Geometry: final body of the model. Coordinates: model frame, mm. Round coordinates to 2 decimals unless told otherwise and drop trailing zeros. Write each loop counter-clockwise with the first axis right and the second up, starting at its lowest first coordinate (ties: lowest second). Pieces come first, ordered by that corner, then holes. Notation, with made-up numbers: M 81.5,78.5 L 88.5,78.5 A34 ccw 88.5,117.5 Z; hole C -38,-33.5 d5. An arc over 180 degrees is marked long. Use one line per item in the form item = value. Start each with the question number.
from build123d import *

# Parameters (mm, degrees)
SKETCH1_R           = 1.5
SKETCH1_R_2         = 2
SKETCH1_W           = 10
SKETCH1_H           = 5
BOSS_EXTRUDE2_DEPTH = 5


with BuildPart() as part:
    # Sketch1 → Boss-Extrude2 (new body)
    with BuildSketch(Plane.XY):
        with BuildLine():
            Line((-126.904376013, 20), (173.095623987, 20))
            ThreePointArc((173.095623987, 20), (193.095623987, 0), (173.095623987, -20))
            Line((173.095623987, -20), (-126.904376013, -20))
            ThreePointArc((-126.904376013, -20), (-146.904376013, 0), (-126.904376013, 20))
        make_face()
        with Locations((-126.904376013, 0)):
            Circle(SKETCH1_R, mode=Mode.SUBTRACT)
        with Locations((173.095623987, 0)):
            Circle(SKETCH1_R_2, mode=Mode.SUBTRACT)
        with Locations((-26.904376013, 0)):
            Circle(SKETCH1_R, mode=Mode.SUBTRACT)
        with Locations((28.095623987, 12.5)):
            Rectangle(SKETCH1_W, SKETCH1_H, mode=Mode.SUBTRACT)
        with Locations((68.095623987, 12.5)):
            Rectangle(SKETCH1_W, SKETCH1_H, mode=Mode.SUBTRACT)
        with Locations((88.095623987, 7.5)):
            Rectangle(SKETCH1_W, SKETCH1_H, mode=Mode.SUBTRACT)
        with Locations((128.095623987, 7.5)):
            Rectangle(SKETCH1_W, SKETCH1_H, mode=Mode.SUBTRACT)
        with Locations((28.095623987, -12.5)):
            Rectangle(SKETCH1_W, SKETCH1_H, mode=Mode.SUBTRACT)
        with Locations((68.095623987, -12.5)):
            Rectangle(SKETCH1_W, SKETCH1_H, mode=Mode.SUBTRACT)
        with Locations((88.095623987, -7.5)):
            Rectangle(SKETCH1_W, SKETCH1_H, mode=Mode.SUBTRACT)
        with Locations((128.095623987, -7.5)):
            Rectangle(SKETCH1_W, SKETCH1_H, mode=Mode.SUBTRACT)
    extrude(amount=BOSS_EXTRUDE2_DEPTH)


solid = part.part
1. Ray query, probe 1 along Y at (x, z) = (126, 3.3); probe 2 along X at (y, z) = (-11, 1); probe 3 along X at (y, z) = (-1, 1.2). Return the intervals inside material, ascending.
2. Contact query for flat-ended pins moving along their axis: pin 1 (1.5 mm diameter, centred on y = -3.5, z = 2.5, fed in from -X); pin 2 (2 mm diameter, centred on y = -15, z = 2.5, fed in from +X); pin 3 (1.5 mm diameter, centred on y = 7.5, z = 3.5, fed in from -X). Output: stop coordinate, or through.
3. Section query A-A (x = 68). Return loops of the section in (y, z).
Checks:
q1.probe_1 = -20 to -10, -5 to 5, 10 to 20
q1.probe_2 = -143.61 to 23.1, 33.1 to 63.1, 73.1 to 189.8
q1.probe_3 = -146.88 to -128.02, -125.79 to -28.02, -25.79 to 171.36, 174.83 to 193.07
q2.pin_1 = -146.71
q2.pin_2 = 187.38
q2.pin_3 = -145.73
q3.outline = M -20,0 L -15,0 L -15,5 L -20,5 Z; M -10,0 L 10,0 L 10,5 L -10,5 Z; M 15,0 L 20,0 L 20,5 L 15,5 Z
